```python
from build123d import *

# Parameters (mm, degrees)
BOSS_EXTRUDE1_DEPTH                              = 38.1
SKETCH2_R                                        = 15.875
SKETCH2_R_2                                      = 6.35
BOSS_EXTRUDE2_DEPTH                              = 7.62
BOSS_EXTRUDE3_DEPTH                              = 6.35
FILLET1_R                                        = 12.7
CSK_FOR_1_4_FLAT_HEAD_MACHINE_SCREW1_D           = 6.7564
CSK_FOR_1_4_FLAT_HEAD_MACHINE_SCREW1_CSINK_D     = 12.8778
CSK_FOR_1_4_FLAT_HEAD_MACHINE_SCREW1_CSINK_ANGLE = 82


with BuildPart() as part:
    # Sketch1 → Boss-Extrude1 (new, symmetric)
    with BuildSketch(Plane.XY):
        Polygon((0, 0), (-34.925, 0), (-34.925, 12.7), (-6.35, 12.7), (-6.35, 6.35), (0, 6.35), align=None)
    extrude(amount=BOSS_EXTRUDE1_DEPTH, both=True)

    # Sketch2 → Boss-Extrude2 (add)
    # profile 1 of 2: a face of its own
    with BuildSketch(Plane(origin=(-6.35, 0, 0), x_dir=(0, 0, -1), z_dir=(1, 0, 0))):
        with BuildLine():
            ThreePointArc((15.875, 63.5), (0, 47.625), (-15.875, 63.5))
            Line((-15.875, 63.5), (-15.875, 12.7))
            Line((-15.875, 12.7), (15.875, 12.7))
            Line((15.875, 12.7), (15.875, 63.5))
        make_face()
    # profile 2 of 2: a face of its own
    with BuildSketch(Plane(origin=(-6.35, 0, 0), x_dir=(0, 0, -1), z_dir=(1, 0, 0))):
        with Locations((0, 63.5)):
            Circle(SKETCH2_R)
        with Locations(Location((0, 63.5, 0), (0, 0, 90))):
            Circle(SKETCH2_R_2, mode=Mode.SUBTRACT)
    extrude(amount=-BOSS_EXTRUDE2_DEPTH)

    # Sketch7 → Boss-Extrude3 (add, symmetric)
    with BuildSketch(Plane.XY):
        Polygon((-13.97, 44.45), (-13.97, 12.7), (-34.925, 12.7), align=None)
    extrude(amount=BOSS_EXTRUDE3_DEPTH, both=True)

    # Fillet1
    fillet1_edges = [part.edges().sort_by_distance(p)[0] for p in [
        (-34.925, 6.35, 38.1),
        (-34.925, 6.35, -38.1),
    ]]
    fillet(fillet1_edges, radius=FILLET1_R)

    # CSK for 1/4 Flat Head Machine Screw1 (through all)
    with Locations(Plane(origin=(0, 12.7, 0), x_dir=(1, 0, 0), z_dir=(0, 1, 0))):
        with Locations((-22.352, 25.4), (-22.352, -25.4)):
            CounterSinkHole(CSK_FOR_1_4_FLAT_HEAD_MACHINE_SCREW1_D / 2, CSK_FOR_1_4_FLAT_HEAD_MACHINE_SCREW1_CSINK_D / 2, counter_sink_angle=CSK_FOR_1_4_FLAT_HEAD_MACHINE_SCREW1_CSINK_ANGLE)


solid = part.part
```
Input: part model. Units: mm. Frame: model coordinates. A direction names the side the tool comes from. Round coordinates to 2 decimals unless told otherwise and drop trailing zeros. Write each loop counter-clockwise with the first axis right and the second up, starting at its lowest first coordinate (ties: lowest second). Pieces come first, ordered by that corner, then holes. Notation, with made-up numbers: M 11,-23 L 51,-23 A15 cw 51,-15 Z; hole C -9.5,-9.75 d10. An arc over 180 degrees is marked long. Write each question's results on one line, items separated by ' | '.
Q1. Section query D-D (y = 18). Return loops of the section in (x, z) (3 decimals).
Results:
outline: M -31.427,-6.35 L -13.97,-6.35 L -13.97,-15.875 L -6.35,-15.875 L -6.35,15.875 L -13.97,15.875 L -13.97,6.35 L -31.427,6.35 Z
Q2. Section query C-C (z = -10.5). Return loops of the section in (x, y) (3 decimals).
Results:
outline: M -34.925,0 L 0,0 L 0,6.35 L -6.35,6.35 L -6.35,75.407 L -13.97,75.407 L -13.97,12.7 L -34.925,12.7 Z
Q3. Section query B-B (y = 50.5). Return loops of the section in (x, z) (3 decimals).
Results:
outline: M -13.97,-15.875 L -6.35,-15.875 L -6.35,15.875 L -13.97,15.875 Z
Q4. Pin query (flat end, axial travel): P1, Ø10.5, axis at x = -27, y = 28.5, coming from the +Z side; P2, Ø12, axis at y = 34, z = 13.5, coming from the +X side; P3, Ø1.5, axis at x = -20, z = 3, coming from the +Y side. Return the tip coordinate at first contact, or that it passes through.
Results:
P1: stops at z = 6.35 | P2: stops at x = -6.35 | P3: stops at y = 36.45
Q5. Access query for faces 1 (the face through (-20, 22, 6.35)), 2 (the face through (-3, 6.35, 1)), 3 (the face through (-10, 38, 15.875)). Directions: +Z, -Z, +X, -X, +Y, -Y. A direction counts if a zero-diameter tool reaches every point of the face in a straight line with its end or side. Return the directions, or none.
Results:
face 1: +Z, -X, +Y | face 2: +Z, -Z, +X, +Y | face 3: +Z, +X, -X, +Y
Q6. Line query: line 1 along X through (y, z) = (2, -25) (3 decimals); line 2 along Z through (x, y) = (-8.25, 63.5) (3 decimals); line 3 along Z through (x, y) = (-25, 7). Output: solid intervals per line, ascending.
Results:
line 1: x = -34.925 to -25.706, -18.998 to 0 | line 2: z = -15.875 to -6.35, 6.35 to 15.875 | line 3: z = -37.79 to -27.5, -23.3 to 23.3, 27.5 to 37.79
Q7. Draft query along X for faces 4 (the face through (-13, 6, 38.1)), 5 (the face through (-19.671, 4.525, 27.456)), 6 (the face through (-34.925, 6, 0)). Return one class per face: released by +X, released by -X, zero draft, split by the parting line, or undercut.
Results:
face 4: zero draft | face 5: undercut | face 6: released by -X
Q8. Section query A-A (z = 0). Return loops of the section in (x, y) (3 decimals), and give its area (3 significant figures).
Results:
outline: M -34.925,0 L 0,0 L 0,6.35 L -6.35,6.35 L -6.35,57.15 L -13.97,57.15 L -13.97,44.45 L -34.925,12.7 Z; M -13.97,69.85 L -6.35,69.85 L -6.35,79.375 L -13.97,79.375 Z | area: 1,150 mm^2
